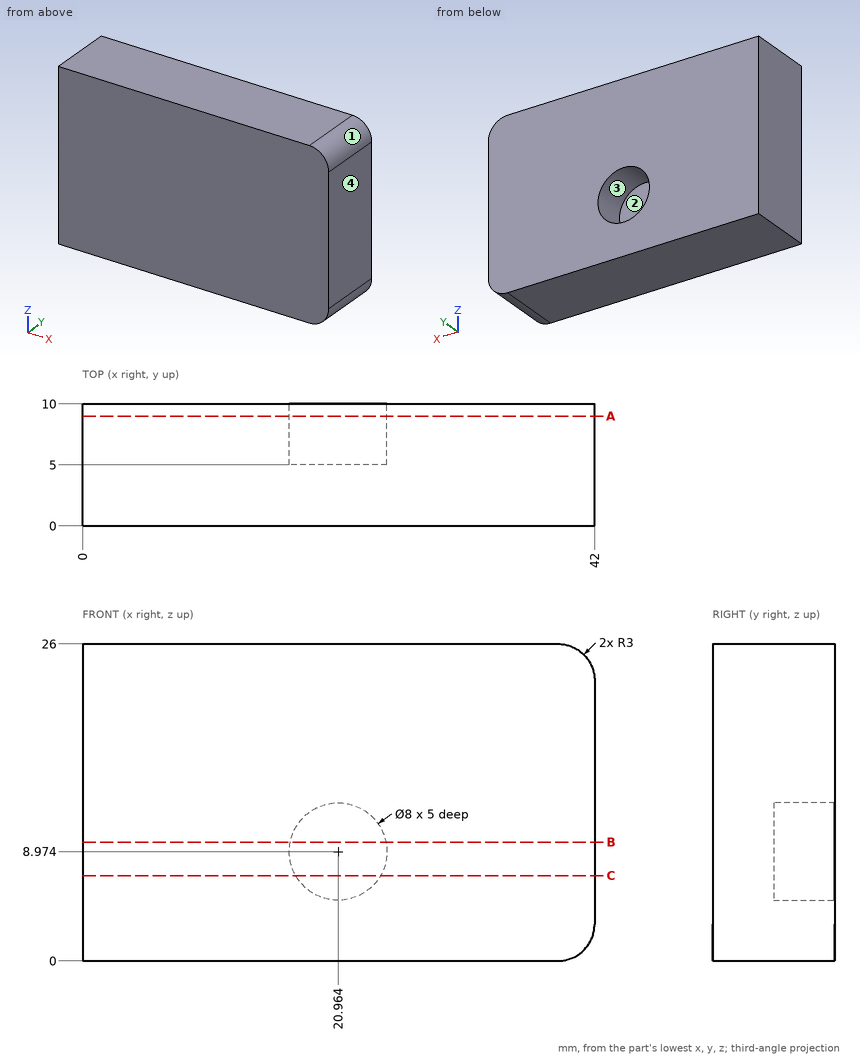
Can you work these out from the drawing? Everything is in mm from the part's minimum corner. Round coordinates to 2 decimals unless told otherwise and drop trailing zeros. Order: outer loops, then holes, each group sorted by start corner. A loop starts at its lowest first (then second) coordinate and runs counter-clockwise, first axis right, second up. Notation, with made-up numbers: M 52,30.5 L 60,30.5 A10 cw 60,40.5 Z; hole C 13.25,59.5 d9. An arc over 180 degrees is marked long. One line per question, with ' | ' between items.
1) For pin 1 Ø3 at (y, z) = (7.5, 18.5) entering from -X, with a flat end and sliding along its axis, tell me the tip position at first contact or that it passes through.
Working result:
pin 1: x = 0
2) I want a section at B-B, the plane z = 9.75. Write out the boundary of the cut face in (x, y).
Working result:
outline: M 0,0 L 42,0 L 42,10 L 24.89,10 L 24.89,5 L 17.04,5 L 17.04,10 L 0,10 Z
3) I want a section at A-A, the plane y = 9. Write out the boundary of the cut face in (x, z) (1 decimal), then the cut area to 3 significant figures.
Working result:
outline: M 0,0 L 39,0 A3 ccw 42,3 L 42,23 A3 ccw 39,26 L 0,26 Z; hole C 21,9 d8 | area: 1,040 mm²
4) I want a section at C-C, the plane z = 7. Write out the boundary of the cut face in (x, y) (1 decimal), then the cut area to 3 significant figures.
Working result:
outline: M 0,0 L 42,0 L 42,10 L 24.4,10 L 24.4,5 L 17.5,5 L 17.5,10 L 0,10 Z | area: 385 mm²
5) I need wall thicknesses on line 1 along Y through (x, z) = (20.5, 8.75); line 2 along X through (y, z) = (5.25, 8) (1 decimal); line 3 along X through (y, z) = (8.75, 7) (1 decimal). Which ranges of each line are inside material? Lowest first, please.
Working result:
line 1: 0 to 5 | line 2: 0 to 17.1, 24.8 to 42 | line 3: 0 to 17.5, 24.4 to 42
6) If we mould it in two halves opening along Z, with no side actions, what happens to the marked faces 1, 2, 3 and 4? For each: +Z half, -Z half, draft (parallel to the pull), parting line (faces both ways), or undercut.
Working result:
face 1: +Z half | face 2: undercut | face 3: undercut | face 4: draft
